Work out the finished part from the listing and answer in its coordinate system (mm). A direction names the side the tool comes from. Coordinates: 2 decimals unless noted, no trailing zeros. Loops run counter-clockwise (first coordinate to the right, second up) from the corner with the lowest first, then second, coordinate; pieces in that order, holes last.
Autodesk Inventor part; units mm, degrees
ref_plane "YZ Plane" through (0, 0, 0) normal (1, 0, 0) x (0, 1, 0)
ref_plane "XZ Plane" through (0, 0, 0) normal (0, 1, 0) x (-1, 0, 0)
ref_plane "XY Plane" through (0, 0, 0) normal (0, 0, 1) x (1, 0, 0)
sketch "Sketch1" plane through (0, 0, 0) normal (0, 0, 1) x (1, 0, 0)
  circle A0 centre (0, 0) radius 10
  circle A1 centre (0, 0) radius 13
  dimension "d0" = 20
  dimension "d1" = 3
extrude "Extrusion1" add sketch "Sketch1" along normal blind 25.2 contours A0 | A1
extrude "Extrusion2" add sketch "Sketch1" against normal blind 17 contours A0
extrude "Extrusion3" add sketch "Sketch1" along normal blind 220 contours A0
properties part number "Axle1" material "Aluminum 6061"
1. A cutting plane is placed at C-C, the plane z = 85.5. Give the vertices of the cut face in (x, y).
2. Each of these flat-tipped pins is pushed along its axis until it touches: P1, Ø2, axis at y = 5, z = 144.5, coming from the -X side; P2, Ø8, axis at x = 6, z = 38, coming from the +Y side; P3, Ø8, axis at x = -9, z = 80, coming from the +Y side; P4, Ø5, axis at x = 1.5, y = -10, coming from the -Z side. Where does it stop, or does it pass through?
3. A cutting plane is placed at A-A, the plane x = 0. Give the vertices of the cut face in (y, z), then the cut area to 3 significant figures.
4. Determine the mould class of faces 1 (the flat face through (7, -8, 0)), 2 (the cylindrical face through (-10.316, 7.91, 12.424)) for opening direction X: released by +X, released by -X, zero draft, split by the parting line, or undercut.
5. For faces 3 (the flat face through (7, -8, 25.2)), 4 (the cylindrical face through (-2.17, -9.76, -8.38)), 5 (the flat face through (0, 0, 220)), determine the directions among +Z, -Z, +X, -X, +Y, -Y from which every point of the face is accessible in a straight line to the end or side of a thin tool.
6. Straight lines are drawn through the part: probe 1 along Z at (x, y) = (10.75, 4); probe 2 along Y at (x, z) = (11.25, 20.5); probe 3 along X at (y, z) = (1, 181.5). For each, find the intervals that lie inside material, in ascending order.
Answers below:
1. outline: circle Ø20 at (0, 0)
2. P1: stops at x = -9.17
2. P2: stops at y = 9.8
2. P3: stops at y = 8.66
2. P4: stops at z = -17
3. outline: (-13, 0) - (-10, 0) - (-10, -17) - (10, -17) - (10, 0) - (13, 0) - (13, 25.2) - (10, 25.2) - (10, 220) - (-10, 220) - (-10, 25.2) - (-13, 25.2) - close
3. area: 4,890 mm2
4. face 1: zero draft
4. face 2: split by the parting line
5. face 3: +Z
5. face 4: -Z
5. face 5: +Z, +X, -X, +Y, -Y
6. probe 1: z = 0 to 25.2
6. probe 2: y = -6.51 to 6.51
6. probe 3: x = -9.95 to 9.95
